The model under review builds one solid part; all positions refer to its coordinate system, in mm. A direction names the side the tool comes from. Round coordinates to 2 decimals unless told otherwise and drop trailing zeros. Order: outer loops, then holes, each group sorted by start corner. A loop starts at its lowest first (then second) coordinate and runs counter-clockwise, first axis right, second up. Notation, with made-up numbers: M 17,83 L 59,83 A14 cw 59,93 Z; hole C -5.5,-23 d2. An arc over 180 degrees is marked long. Answer as a JSON object with one key per item and string values. Group by question number.
1. Clearance check with flat-ended pins moving along their axes: P1, Ø3, axis at x = -0.5, z = -5.5, coming from the +Y side; P2, Ø2, axis at x = -1, z = 5.5, coming from the -Y side; P3, Ø2.5, axis at y = 0.5, z = 11.5, coming from the -X side; P4, Ø1, axis at y = 0, z = 0, coming from the +X side. State where each tip first meets the part, or that it passes through.
2. Machinability: for faces 1 (the face through (-1, 3, 7.5)), 2 (the face through (3.612, -3.312, 9.972)), 3 (the face through (-1.233, 2.175, 11.021)), which of the approach directions +Z, -Z, +X, -X, +Y, -Y give a long, thin tool a straight path to every point of the face, cutting with its end or side? Answer none if there is none.
3. Add section B-B on z = 9. State the section outline as (x, y) points.
4. To check wall thickness, follow probe 1 along Z at (x, y) = (1, -1); probe 2 along Z at (x, y) = (-2, -2.75); probe 3 along X at (y, z) = (-0.5, 11.5). State the ranges of each line that lie inside material, in increasing order. Write a range as [from, to].
5. Add section A-A on z = -8. State the section outline as (x, y) points, and give its area (3 significant figures).
6. Mouldability with a two-part tool opening along Y and no side actions: class faces 4 (the face through (1.267, 2.155, 11.021)), 5 (the face through (-2.86, -0.9, -2.39)), 6 (the face through (2, -2, 12.5)) as released by +Y, released by -Y, zero draft, split by the parting line, or undercut.
```python
from build123d import *

# Parameters (mm, degrees)
FILLET_1_R          = 0.5
FILLET_2_SIZE       = 0.5
FILLET_2_SIZE_2     = 0.8
CHAMFER_1_SIZE      = 0.5
CHAMFER_1_SIZE2     = 0.866025404
CUT_EXTRUDE_1_DEPTH = 3


with BuildPart() as part:
    # 草图2 → 旋转1 (revolve)
    with BuildSketch(Plane(origin=(0, 0, 0), x_dir=(0, 0, -1), z_dir=(1, 0, 0)), mode=Mode.PRIVATE) as revolve_1_sk:
        Polygon((-12.5, 0), (-12.5, 4.9), (-7.5, 4.9), (-7.5, 3), (12.5, 3), (12.5, 0), align=None)
    revolve(revolve_1_sk.sketch.rotate(Axis((0, 0, -12.5), (0, 0, 1)), 90), axis=Axis((0, 0, -12.5), (0, 0, 1)))

    # 圆角1
    fillet_1_edges = [part.edges().sort_by_distance(p)[0] for p in [
        (4.9, 0, 7.5),
    ]]
    fillet(fillet_1_edges, radius=FILLET_1_R)

    # 圆角2
    # an asymmetric fillet: 0.8, 0.5 mm, written as the material it takes off along each edge
    with BuildSketch(Plane(origin=(0, 0, 12.5), x_dir=(-1, 0, 0), z_dir=(0, 1, 0))) as fillet_2_piece_1:
        with BuildLine():
            Bezier((4.9, -FILLET_2_SIZE), (4.9, 0), (4.9 - FILLET_2_SIZE_2, 0), weights=[1, 0.707106781, 1])
            Line((4.9 - FILLET_2_SIZE_2, 0), (4.9, 0))
            Line((4.9, 0), (4.9, -FILLET_2_SIZE))
        make_face()
    revolve(axis=Axis((0, 0, 12.5), (0, 0, 1)), mode=Mode.SUBTRACT)

    # 倒角1
    chamfer_1_edges = [part.edges().sort_by_distance(p)[0] for p in [
        (3, 0, -12.5),
    ]]
    chamfer_1_side = [part.faces().sort_by_distance(p)[0] for p in [
        (3, 0, -2.5),
    ]]
    chamfer(chamfer_1_edges, length=CHAMFER_1_SIZE, length2=CHAMFER_1_SIZE2, reference=chamfer_1_side[0])

    # 草图3 → 切除-拉伸1 (cut)
    with BuildSketch(Plane.XY.offset(12.5)):
        Polygon((0, 2.886751346), (-2.5, 1.443375673), (-2.5, -1.443375673), (0, -2.886751346), (2.5, -1.443375673), (2.5, 1.443375673), align=None)
    extrude(amount=-CUT_EXTRUDE_1_DEPTH, mode=Mode.SUBTRACT)


solid = part.part
```
Recorded:
{
 "1": {"P1": "stops at y = 3", "P2": "stops at y = -3", "P3": "stops at x = -4.9", "P4": "stops at x = 3"},
 "2": {"face 1": "-Z", "face 2": "+Z, -Z", "face 3": "+Z"},
 "3": {"outline": "C 0,0 d9.8"},
 "4": {"probe 1": "z = [-12.5, 9.5]", "probe 2": "z = [7.5, 12.5]", "probe 3": "x = [-4.87, -2.5], [2.5, 4.87]"},
 "5": {"outline": "C 0,0 d6", "area": "28.3 mm²"},
 "6": {"face 4": "undercut", "face 5": "split by the parting line", "face 6": "zero draft"}
}
